from build123d import *
from OCP.BRepFilletAPI import BRepFilletAPI_MakeChamfer

# Parameters (mm, degrees)
BOSS_EXTRUDE1_DEPTH = 3
CHAMFER1_SIZE       = 3
CHAMFER1_SIZE_2     = 1.853922924
CUT_EXTRUDE1_DEPTH  = 10
SKETCH2_R           = 2
CUT_EXTRUDE2_DEPTH  = 1.5
SKETCH5_R           = 2
CUT_EXTRUDE3_DEPTH  = 1.5
SKETCH9_R           = 2
CUT_EXTRUDE4_DEPTH  = 1.5
SKETCH10_R          = 2
CUT_EXTRUDE5_DEPTH  = 1.5
SKETCH11_R          = 2
CUT_EXTRUDE6_DEPTH  = 1.5


with BuildPart() as part:
    # Sketch1 → Boss-Extrude1 (new body)
    with BuildSketch(Plane(origin=(0, 0, 0), x_dir=(1, 0, 0), z_dir=(0, 1, 0))):
        Polygon((92.27247452, 0), (28.51376274, 87.756338167), (-74.65, 54.236399716), (-74.65, -54.236399716), (28.51376274, -87.756338167), align=None)
    extrude(amount=BOSS_EXTRUDE1_DEPTH)

    # Chamfer1
    chamfer1_edges_1 = [part.edges().sort_by_distance(p)[0] for p in [
        (-74.65, 3, 0),
    ]]
    chamfer1_side_1 = [part.faces().sort_by_distance(p)[0] for p in [
        (-74.65, 2.962921542, 0),
    ]]
    chamfer1_edges_2 = [part.edges().sort_by_distance(p)[0] for p in [
        (-23.06811863, 3, -70.996368941),
    ]]
    chamfer1_side_2 = [part.faces().sort_by_distance(p)[0] for p in [
        (-23.06811863, 2.962921542, -70.996368941),
    ]]
    chamfer1_edges_3 = [part.edges().sort_by_distance(p)[0] for p in [
        (60.39311863, 3, -43.878169084),
    ]]
    chamfer1_side_3 = [part.faces().sort_by_distance(p)[0] for p in [
        (60.39311863, 2.962921542, -43.878169084),
    ]]
    chamfer1_edges_4 = [part.edges().sort_by_distance(p)[0] for p in [
        (60.39311863, 3, 43.878169084),
    ]]
    chamfer1_side_4 = [part.faces().sort_by_distance(p)[0] for p in [
        (60.39311863, 2.962921542, 43.878169084),
    ]]
    chamfer1_edges_5 = [part.edges().sort_by_distance(p)[0] for p in [
        (-23.06811863, 3, 70.996368941),
    ]]
    chamfer1_side_5 = [part.faces().sort_by_distance(p)[0] for p in [
        (-23.06811863, 2.962921542, 70.996368941),
    ]]
    chamfer1 = BRepFilletAPI_MakeChamfer(part.part.solid().wrapped)
    for e in chamfer1_edges_1:
        chamfer1.Add(CHAMFER1_SIZE - 0.0001, CHAMFER1_SIZE_2 - 0.0001, e.wrapped, chamfer1_side_1[0].wrapped)
    for e in chamfer1_edges_2:
        chamfer1.Add(CHAMFER1_SIZE - 0.0001, CHAMFER1_SIZE_2 - 0.0001, e.wrapped, chamfer1_side_2[0].wrapped)
    for e in chamfer1_edges_3:
        chamfer1.Add(CHAMFER1_SIZE - 0.0001, CHAMFER1_SIZE_2 - 0.0001, e.wrapped, chamfer1_side_3[0].wrapped)
    for e in chamfer1_edges_4:
        chamfer1.Add(CHAMFER1_SIZE - 0.0001, CHAMFER1_SIZE_2 - 0.0001, e.wrapped, chamfer1_side_4[0].wrapped)
    for e in chamfer1_edges_5:
        chamfer1.Add(CHAMFER1_SIZE - 0.0001, CHAMFER1_SIZE_2 - 0.0001, e.wrapped, chamfer1_side_5[0].wrapped)
    add(Compound.cast(chamfer1.Shape()), mode=Mode.REPLACE)  # a hair under: the kernel refuses the full size

    # 3DSketch1 → Cut-Extrude1 (cut)
    with BuildSketch(Plane(origin=(-58.35, 0, -42.393756509), x_dir=(0.9510565162951536, 0, 0.3090169943749475), z_dir=(0, -1, 0))):
        Polygon((0, 0), (26.200782433, 80.637716756), (110.988295452, 80.637716756), (137.189077885, 0), (68.594538943, -49.836849731), align=None)
    extrude(amount=-CUT_EXTRUDE1_DEPTH, mode=Mode.SUBTRACT)

    # Sketch2 → Cut-Extrude2 (cut, along a direction that is not the sketch's normal)
    with BuildSketch(Plane(origin=(0, 3, 0), x_dir=(1, 0, 0), z_dir=(0, 1, 0))):
        with Locations((-67.132958116, 48.774949102)):
            Circle(SKETCH2_R)
    extrude(amount=-CUT_EXTRUDE2_DEPTH, dir=(0.4910935234360901, 0.7946827516361096, 0.3568003300043147), mode=Mode.SUBTRACT)

    # Sketch5 → Cut-Extrude3 (cut, along a direction that is not the sketch's normal)
    with BuildSketch(Plane(origin=(0, 3, 0), x_dir=(1, 0, 0), z_dir=(0, 1, 0))):
        with Locations((25.642508235, 78.919525446)):
            Circle(SKETCH5_R)
    extrude(amount=-CUT_EXTRUDE3_DEPTH, dir=(-0.1875810342976446, 0.7946827516361096, 0.577315061144162), mode=Mode.SUBTRACT)

    # Sketch9 → Cut-Extrude4 (cut, along a direction that is not the sketch's normal)
    with BuildSketch(Plane(origin=(0, 3, 0), x_dir=(1, 0, 0), z_dir=(0, 1, 0))):
        with Locations((82.980899762, 0)):
            Circle(SKETCH9_R)
    extrude(amount=-CUT_EXTRUDE4_DEPTH, dir=(-0.6070249782768915, 0.7946827516361101, 3.1127032543975076e-15), mode=Mode.SUBTRACT)

    # Sketch10 → Cut-Extrude5 (cut, along a direction that is not the sketch's normal)
    with BuildSketch(Plane(origin=(0, 3, 0), x_dir=(1, 0, 0), z_dir=(0, 1, 0))):
        with Locations((25.642508235, -78.919525446)):
            Circle(SKETCH10_R)
    extrude(amount=-CUT_EXTRUDE5_DEPTH, dir=(-0.18758103429764075, 0.7946827516361107, -0.5773150611441616), mode=Mode.SUBTRACT)

    # Sketch11 → Cut-Extrude6 (cut, along a direction that is not the sketch's normal)
    with BuildSketch(Plane(origin=(0, 3, 0), x_dir=(1, 0, 0), z_dir=(0, 1, 0))):
        with Locations((-67.132958116, -48.774949102)):
            Circle(SKETCH11_R)
    extrude(amount=-CUT_EXTRUDE6_DEPTH, dir=(0.49109352343609003, 0.7946827516361095, -0.35680033000431516), mode=Mode.SUBTRACT)


solid = part.part
Part model, mm, in its own coordinate system. A direction names the side the tool comes from. Coordinates: 2 decimals unless noted, no trailing zeros. Loops run counter-clockwise (first coordinate to the right, second up) from the corner with the lowest first, then second, coordinate; pieces in that order, holes last. Notation, with made-up numbers: M -32.5,88.25 L 24.5,88.25 A14 cw 24.5,98.25 Z; hole C 35.25,6 d11. An arc over 180 degrees is marked long. Use a Markdown table: item, result. Add a question column.
Q1. Which spindle directions (+Z, -Z, +X, -X, +Y, -Y) get a long thin tool onto all of the face, cutting with end or side? Do faces 5 (the flat face through (-23.5, 1.52, 69.87)), 6 (the flat face through (26, 1.808, -80)), 7 (the flat face through (-17.467, 1.479, -55.678)). Say none if no direction does.
Q2. Probe L1, parallel to Z at x = 35.5, y = 2.6; L2, parallel to Z at x = 16, y = 2.8; L3, parallel to X at y = 1.8, z = -12.5. List the from-to ranges inside material, lowest first.
Q3. Pin check, flat tips, straight feed: P1, Ø1.5, axis at x = 46.5, y = 1.5, coming from the +Z side; P2, Ø1.5, axis at x = 36, y = 2.5, coming from the +Z side; P3, Ø1.2, axis at x = 83.5, z = 0, coming from the +Y side. Stop position of each tip, or through.
Q4. Mould opens along Z. For faces 1 (the flat face through (59.19, 1.52, 43.94)), 2 (the flat face through (-22.056, 1.521, -70.337)), 3 (the flat face through (26, 1.808, 80)), 4 (the flat face through (44.39, 3, -38.43)) say: +Z half, -Z half, draft (parallel to the pull), parting line (faces both ways), or undercut.
Q5. Cut at C-C (y = 0.8). Write the cut outline in (x, z), and give its area (3 significant figures).
Worked out:
| question | item | result |
|---|---|---|
| 1 | face 5 | +Z, -X, +Y |
| 1 | face 6 | none |
| 1 | face 7 | +Y, -Y |
| 2 | L1 | z = -75.41 to -50.41, 50.41 to 75.41 |
| 2 | L2 | z = -81.87 to -66.55, 66.55 to 81.87 |
| 2 | L3 | x = -73.54 to -58.35, 63.04 to 81.82 |
| 3 | P1 | stops at z = 62.72 |
| 3 | P2 | stops at z = 76.12 |
| 3 | P3 | stops at y = 1.81 |
| 4 | face 1 | +Z half |
| 4 | face 2 | -Z half |
| 4 | face 3 | undercut |
| 4 | face 4 | draft |
| 5 | outline | M -74.16,-53.88 L 28.32,-87.18 L 91.66,0 L 28.32,87.18 L -74.16,53.88 Z; hole M -58.35,-42.39 L 22.29,-68.59 L 72.12,0 L 22.29,68.59 L -58.35,42.39 Z |
| 5 | area | 7,610 mm2 |
